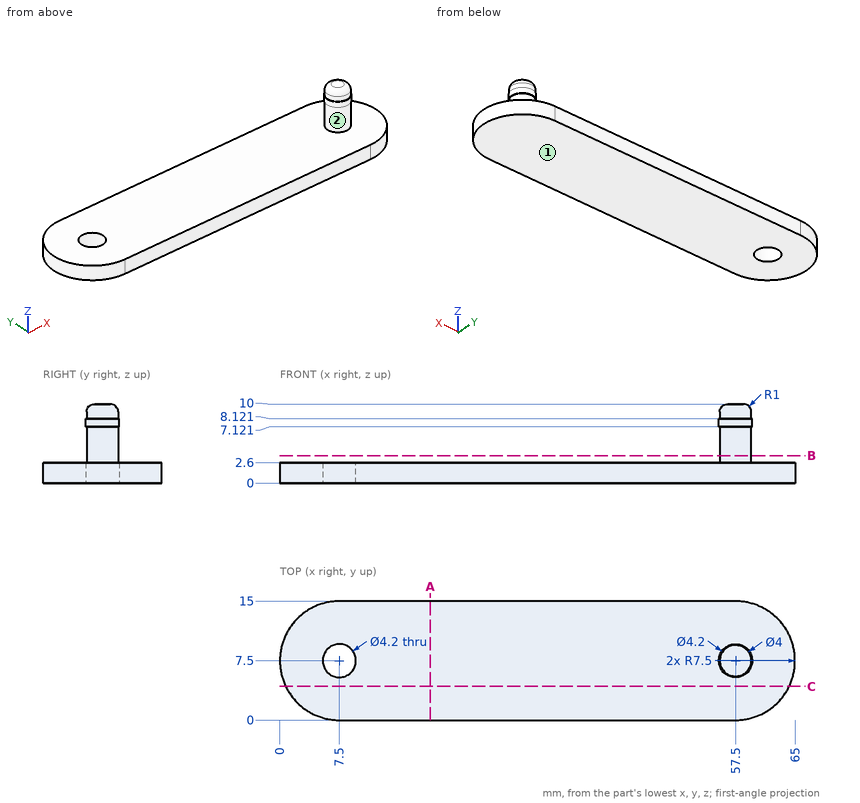
Input: dimensioned drawing with shaded views. Units: mm. Origin: part minimum x, y, z. Coordinates: 2 decimals unless noted, no trailing zeros. Loops run counter-clockwise (first coordinate to the right, second up) from the corner with the lowest first, then second, coordinate; pieces in that order, holes last. Notation, with made-up numbers: M -30.5,-12.5 L 15.5,-12.5 A10 cw 15.5,-6.5 Z; hole C 89.25,87.25 d9. An arc over 180 degrees is marked long. One line per item, written item: value. Start each with the question number.
1) Pin query (flat end, axial travel): P1, Ø3, axis at y = 10.5, z = 3.5, coming from the +X side; P2, Ø2, axis at x = 23, y = 11, coming from the +Z side; P3, Ø2, axis at y = 11, z = 5, coming from the +X side; P4, Ø4, axis at x = 56.5, z = 5.5, coming from the +Y side. Return the tip coordinate at first contact, or that it passes through.
2) Draft query along Z for the marked faces 1 and 2. Return one class per face: released by +Z, released by -Z, zero draft, split by the parting line, or undercut.
3) Cut plane C-C (y = 4.25). Return loops of the section in (x, z), then the cut area to 3 significant figures.
4) Cut plane A-A (x = 19). Return loops of the section in (y, z).
5) Material intervals for L1, parallel to Z at x = 56, y = 13.5; L2, parallel to Y at x = 7.5, z = 1.3; L3, parallel to X at y = 6.5, z = 2, sorted ascending. Write a range as from..to.
6) Cut plane B-B (z = 3.5). Return loops of the section in (x, y).
Evaluation:
1. P1: x = 64.78
1. P2: z = 2.6
1. P3: through
1. P4: y = 9.6
2. face 1: released by -Z
2. face 2: undercut
3. outline: M 0.74,0 L 64.26,0 L 64.26,2.6 L 0.74,2.6 Z
3. area: 165 mm^2
4. outline: M 0,0 L 15,0 L 15,2.6 L 0,2.6 Z
5. L1: 0..2.6
5. L2: 0..5.4, 9.6..15
5. L3: 0.07..5.65, 9.35..64.93
6. outline: C 57.5,7.5 d4
